Read the model definition and answer for the solid it produces. Units are mm, in the model's axes. Round coordinates to 2 decimals unless told otherwise and drop trailing zeros. Loops run counter-clockwise (first coordinate to the right, second up) from the corner with the lowest first, then second, coordinate; pieces in that order, holes last. Notation, with made-up numbers: M 20.25,85.5 L 45.25,85.5 A18 ccw 45.25,99.5 Z; hole C 85,-32 d3. An arc over 180 degrees is marked long. Write each question's results on one line, items separated by ' | '.
from build123d import *

# Parameters (mm, degrees)
BOSS_EXTRU_1_DEPTH = 5
CONG_1_R           = 2


with BuildPart() as part:
    # Esquisse1 → Boss.-Extru.1 (new body)
    with BuildSketch(Plane.XY):
        with BuildLine():
            Line((-79.83772234, 0), (-60.16227766, 0))
            ThreePointArc((-60.16227766, 0), (-57, -10), (-53.83772234, 0))
            Line((-53.83772234, 0), (53.83772234, 0))
            ThreePointArc((53.83772234, 0), (57, -10), (60.16227766, 0))
            Line((60.16227766, 0), (79.83772234, 0))
            ThreePointArc((79.83772234, 0), (83, -10), (86.16227766, 0))
            Line((86.16227766, 0), (95, 0))
            Line((95, 0), (95, -15))
            Line((95, -15), (-95, -15))
            Line((-95, -15), (-95, 0))
            Line((-95, 0), (-86.16227766, 0))
            ThreePointArc((-86.16227766, 0), (-83, -10), (-79.83772234, 0))
        make_face()
    extrude(amount=BOSS_EXTRU_1_DEPTH)

    # Congé1
    cong_1_edges = [part.edges().sort_by_distance(p)[0] for p in [
        (-86.16227766, 0, 2.5),
        (-79.83772234, 0, 2.5),
        (-60.16227766, 0, 2.5),
        (-53.83772234, 0, 2.5),
        (53.83772234, 0, 2.5),
        (60.16227766, 0, 2.5),
        (79.83772234, 0, 2.5),
        (86.16227766, 0, 2.5),
        (95, 0, 2.5),
        (95, -15, 2.5),
        (-95, -15, 2.5),
        (-95, 0, 2.5),
    ]]
    fillet(cong_1_edges, radius=CONG_1_R)


solid = part.part
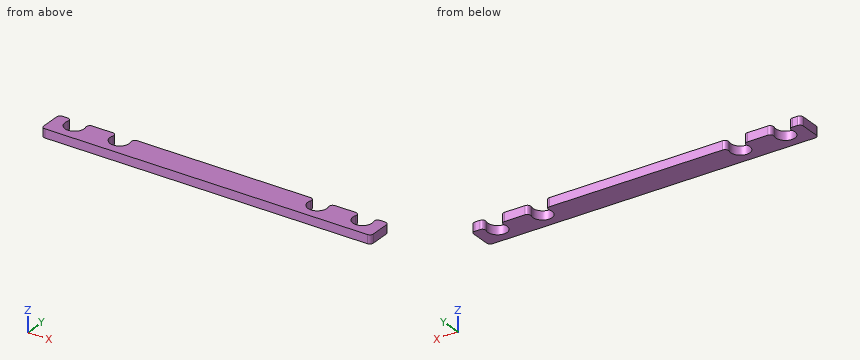
Item 1: Flat-ended cylindrical pins translate along their axes: pin 1 (9 mm diameter, centred on x = 83, y = -4.5, fed in from -Z); pin 2 (1.5 mm diameter, centred on x = 57.5, y = -10.5, fed in from -Z). Find the tip coordinate at first contact, or state that the pin passes through.
Outcome:
pin 1: passes through | pin 2: stops at z = 0
Item 2: The part is cut by section A-A (y = -4.5). Determine the outline of the cut face in (x, z).
Outcome:
outline: M -95,0 L -88.5,0 L -88.5,5 L -95,5 Z; M -77.5,0 L -62.5,0 L -62.5,5 L -77.5,5 Z; M -51.5,0 L 51.5,0 L 51.5,5 L -51.5,5 Z; M 62.5,0 L 77.5,0 L 77.5,5 L 62.5,5 Z; M 88.5,0 L 95,0 L 95,5 L 88.5,5 Z
Item 3: The part is cut by section C-C (z = 4). Determine the outline of the cut face in (x, y).
Outcome:
outline: M -95,-13 A2 ccw -93,-15 L 93,-15 A2 ccw 95,-13 L 95,-2 A2 ccw 93,0 L 90.07,0 A2 ccw 88.19,-2.67 A5.5 cw long 77.81,-2.67 A2 ccw 75.93,0 L 64.07,0 A2 ccw 62.19,-2.67 A5.5 cw long 51.81,-2.67 A2 ccw 49.93,0 L -49.93,0 A2 ccw -51.81,-2.67 A5.5 cw long -62.19,-2.67 A2 ccw -64.07,0 L -75.93,0 A2 ccw -77.81,-2.67 A5.5 cw long -88.19,-2.67 A2 ccw -90.07,0 L -93,0 A2 ccw -95,-2 Z
Item 4: The part is cut by section B-B (x = -57). Determine the outline of the cut face in (y, z), plus the area to 3 significant figures.
Outcome:
outline: M -15,0 L -10,0 L -10,5 L -15,5 Z | area: 25.0 mm2
Item 5: Straight lines are drawn through the part: line 1 (X direction, y = -4.5, z = 3.1); line 2 (X direction, y = -3.25, z = 3.05); line 3 (Y direction, x = -57, z = 3.8). For each, find the intervals that lie inside material, in ascending order.
Outcome:
line 1: x = -95 to -88.5, -77.5 to -62.5, -51.5 to 51.5, 62.5 to 77.5, 88.5 to 95 | line 2: x = -95 to -88.36, -77.64 to -62.36, -51.64 to 51.64, 62.36 to 77.64, 88.36 to 95 | line 3: y = -15 to -10
